For this review, take the finished solid that the model builds, in its own axes (mm). A direction names the side the tool comes from. Round coordinates to 2 decimals unless told otherwise and drop trailing zeros. Write each loop counter-clockwise with the first axis right and the second up, starting at its lowest first coordinate (ties: lowest second). Pieces come first, ordered by that corner, then holes.
from build123d import *

# Parameters (mm, degrees)
SKETCH1_R           = 2.032
SKETCH1_R_2         = 0.80645
SKETCH1_W           = 15.24
SKETCH1_H           = 2.794
BOSS_EXTRUDE1_DEPTH = 2.794


with BuildPart() as part:
    # Sketch1 → Boss-Extrude1 (new body)
    with BuildSketch(Plane(origin=(0, 0, 0), x_dir=(1, 0, 0), z_dir=(0, 1, 0))):
        Polygon((0, 0), (111.5314, 0), (0, 111.5314), align=None)
        with Locations((24.965112017, 26.93738734)):
            Circle(SKETCH1_R, mode=Mode.SUBTRACT)
        with Locations((20.464232017, 26.93738734)):
            Circle(SKETCH1_R_2, mode=Mode.SUBTRACT)
        with Locations((29.465992017, 26.93738734)):
            Circle(SKETCH1_R_2, mode=Mode.SUBTRACT)
        with Locations((26.67, 3.937)):
            Rectangle(SKETCH1_W, SKETCH1_H, mode=Mode.SUBTRACT)
        with Locations((80.01, 3.937)):
            Rectangle(SKETCH1_W, SKETCH1_H, mode=Mode.SUBTRACT)
        Polygon((16.164461018, 91.774836534), (26.940768363, 80.998529188), (24.965112017, 79.022872842), (14.188804671, 89.799180187), align=None, mode=Mode.SUBTRACT)
        Polygon((68.24994652, 39.689351031), (79.026253865, 28.913043686), (77.050597519, 26.93738734), (66.274290173, 37.713694685), align=None, mode=Mode.SUBTRACT)
    extrude(amount=BOSS_EXTRUDE1_DEPTH)


solid = part.part
(1) For pin 1 Ø0.8 at (y, z) = (1.5, -4) entering from +X; pin 2 Ø1.5 at (y, z) = (0.5, -35.5) entering from +X; pin 3 Ø0.8 at (x, y) = (30.5, 2) entering from -Z; pin 4 Ø3.5 at (x, z) = (24.97, -26.94) entering from -Y, all flat-tipped, find the tip position at first contact; note any pin that passes through.
Geometry check:
pin 1: stops at x = 107.93
pin 2: stops at x = 76.78
pin 3: stops at z = -81.43
pin 4: passes through
(2) We need section C-C, the plane z = -34. Give the boundary of the cut face in (x, y), and give its area (3 significant figures).
Geometry check:
outline: (0, 0) - (69.99, 0) - (69.99, 2.79) - (0, 2.79) - close; (73.94, 0) - (77.53, 0) - (77.53, 2.79) - (73.94, 2.79) - close
area: 206 mm2
(3) Mouldability with a two-part tool opening along X and no side actions: class faces 3 (the face through (0, 1, -57)), 4 (the face through (87.63, 1, -4)), 5 (the face through (30, 2.794, -32)) as pulls with the +X half, pulls with the -X half, needs draft (parallel to the pull), parting line crosses it, or undercut.
Geometry check:
face 3: pulls with the -X half
face 4: undercut
face 5: needs draft
(4) For line 1 along Z through (x, y) = (21.5, 1.3); line 2 along Z through (x, y) = (76.5, 0.1); line 3 along Z through (x, y) = (26, 2.65), list the stretches that pass through material, from the lowest coordinate up.
Geometry check:
line 1: z = -90.03 to -86.44, -82.49 to -5.33, -2.54 to 0
line 2: z = -35.03 to -31.44, -27.49 to -5.33, -2.54 to 0
line 3: z = -85.53 to -81.94, -80.06 to -28.69, -25.19 to -5.33, -2.54 to 0
(5) For faces 1 (the face through (30, 0, -32)), 2 (the face through (34.29, 1, -4)), list the 3-axis set-ups (+Z, -Z, +X, -X, +Y, -Y) from which the entire face can be reached by the end or side of a thin tool; tool diameter is ignored.
Geometry check:
face 1: +Z, -Z, +X, -X, -Y
face 2: +Y, -Y
(6) We need section A-A, the plane y = 1.65. Give the boundary of the cut face in (x, z), and give its area (3 significant figures).
Geometry check:
outline: (0, -111.53) - (111.53, 0) - (0, 0) - close; hole (14.19, -89.8) - (16.16, -91.77) - (26.94, -81) - (24.97, -79.02) - close; hole (19.05, -5.33) - (34.29, -5.33) - (34.29, -2.54) - (19.05, -2.54) - close; hole circle Ø1.61 at (20.46, -26.94); hole circle Ø4.06 at (24.97, -26.94); hole circle Ø1.61 at (29.47, -26.94); hole (66.27, -37.71) - (68.25, -39.69) - (79.03, -28.91) - (77.05, -26.94) - close; hole (72.39, -5.33) - (87.63, -5.33) - (87.63, -2.54) - (72.39, -2.54) - close
area: 6,030 mm2
(7) We need section D-D, the plane z = -65. Give the boundary of the cut face in (x, y).
Geometry check:
outline: (0, 0) - (46.53, 0) - (46.53, 2.79) - (0, 2.79) - close
(8) We need section B-B, the plane x = 71. Give the boundary of the cut face in (y, z), and give its area (3 significant figures).
Geometry check:
outline: (0, -40.53) - (2.79, -40.53) - (2.79, -36.94) - (0, -36.94) - close; (0, -32.99) - (2.79, -32.99) - (2.79, 0) - (0, 0) - close
area: 102 mm2
